Input: part model. Units: mm. Frame: model coordinates. Face numbers are marked on the shaded views. A direction names the side the tool comes from. Give positions to 0.01 mm unless a question says otherwise; leave off trailing zeros. Loops run counter-clockwise (first coordinate to the right, second up) from the corner with the lowest first, then second, coordinate; pieces in that order, holes last. Notation, with made-up numbers: M -19.5,-2 L 36.5,-2 A12 ccw 36.5,2 Z; hole C 26,-4.5 d9. An arc over 180 degrees is marked long. Answer as a JSON object with one key per item and string values. Group by question number.
1) Draft query along Z for the marked faces 1, 2, 3 and 4. Return one class per face: +Z half, -Z half, draft (parallel to the pull), parting line (faces both ways), or undercut.
2) Section query C-C on z = 1. Return loops of the section in (x, y), plus the area to 3 significant figures.
3) Section query D-D on y = 1.65. Return loops of the section in (x, z), plus the area to 3 significant figures.
4) Access query for the marked faces 5 and 6. Directions: +Z, -Z, +X, -X, +Y, -Y. A direction counts if a zero-diameter tool reaches every point of the face in a straight line with its end or side. Return the directions, or none.
5) First-contact query: P1, Ø1.5, axis at x = -3.5, y = 0.5, coming from the -Z side. Flat tip, straight axial feed; report the tip coordinate or a pass-through.
6) Section query A-A on x = 0. Return loops of the section in (y, z), plus the area to 3 significant figures.
7) Ray query, L1, parallel to Z at x = 0, y = 0.4; L2, parallel to Z at x = -5.5, y = 0; L3, parallel to X at y = 1.8, z = -32. Return the intervals inside material, ascending.
8) Section query B-B on x = 8.5. Return loops of the section in (y, z).
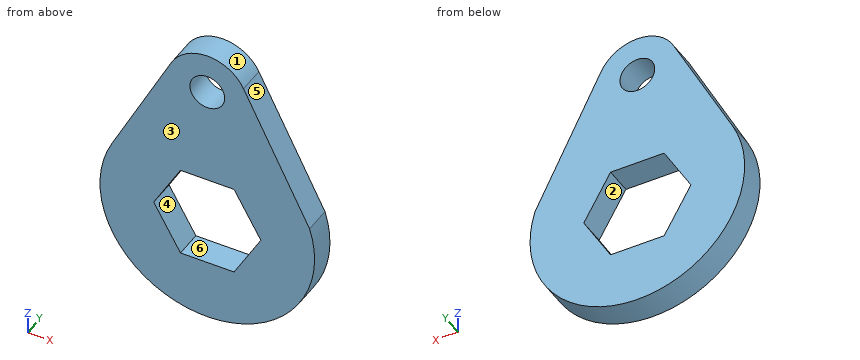
Autodesk Inventor part; units mm, degrees
ref_plane "YZ Plane" through (0, 0, 0) normal (1, 0, 0) x (0, 1, 0)
ref_plane "XZ Plane" through (0, 0, 0) normal (0, 1, 0) x (-1, 0, 0)
ref_plane "XY Plane" through (0, 0, 0) normal (0, 0, 1) x (1, 0, 0)
sketch "Sketch1" plane through (0, 0, 0) normal (0, 1, 0) x (-1, 0, 0)
  circle A0 centre (0, 0) radius 3
  circle A1 centre (0, 0) radius 7
  circle A2 centre (0, -25) radius 18.5
  line L0 (6.2154, 3.22) -> (16.4265, -16.49)
  line L1 (-17.6376, -19.4175) -> (-6.2496, 3.1532)
  line L2 (9.2376, -25) -> (4.6188, -33)
  line L3 (4.6188, -33) -> (-4.6188, -33)
  line L4 (-4.6188, -33) -> (-9.2376, -25)
  line L5 (-9.2376, -25) -> (-4.6188, -17)
  line L6 (-4.6188, -17) -> (4.6188, -17)
  line L7 (4.6188, -17) -> (9.2376, -25)
  point P0 (4.4139, 5.433)
  point P1 (-13.2255, -12.0641)
  dimension "d3" = 6
  dimension "d6" = 14
  dimension "d11" = 25
  dimension "d12" = 37
  dimension "d13" = 16
extrude "Plate1" add sketch "Sketch1" along normal mid plane 4.7 contours A1 A2 | A1 L0 A2 | A2 L1 A1 | A1 A2 | A1 A2 L1
equation "\"d9\" = Thickness"
equation "\"BendRadius\" = Thickness"
equation "\"BendReliefWidth\" = Thickness"
equation "\"BendReliefDepth\" = 0.5 * Thickness"
equation "\"CornerReliefSize\" = 4 * Thickness"
equation "\"MinimumRemnant\" = 2 * Thickness"
equation "\"TransitionRadius\" = BendRadius"
equation "\"JacobiRadiusSize\" = BendRadius"
equation "\"GapSize\" = Thickness"
properties part number "palanca2"
Output:
{
 "1": {"face 1": "+Z half", "face 2": "undercut", "face 3": "draft", "face 4": "undercut"},
 "2": {"outline": "M -7.37,-2.35 L -2.83,-2.35 L -2.83,2.35 L -7.37,2.35 Z; M 2.83,-2.35 L 7.34,-2.35 L 7.34,2.35 L 2.83,2.35 Z", "area": "42.5 mm^2"},
 "3": {"outline": "M -16.43,-16.49 A18.5 ccw long 17.64,-19.42 L 6.25,3.15 A7 ccw -6.22,3.22 Z; hole M -9.24,-25 L -4.62,-33 L 4.62,-33 L 9.24,-25 L 4.62,-17 L -4.62,-17 Z; hole C 0,0 d6", "area": "1,070 mm^2"},
 "4": {"face 5": "+Z, +X, +Y, -Y", "face 6": "+Y, -Y"},
 "5": {"P1": "stops at z = -43.29"},
 "6": {"outline": "M -2.35,-43.5 L 2.35,-43.5 L 2.35,-33 L -2.35,-33 Z; M -2.35,-17 L 2.35,-17 L 2.35,-3 L -2.35,-3 Z; M -2.35,3 L 2.35,3 L 2.35,7 L -2.35,7 Z", "area": "134 mm^2"},
 "7": {"L1": "z = -43.5 to -33, -17 to -3, 3 to 7", "L2": "z = -42.66 to -31.47, -18.53 to 4.33", "L3": "x = -17.12 to -5.2, 5.2 to 17.12"},
 "8": {"outline": "M -2.35,-41.43 L 2.35,-41.43 L 2.35,-26.28 L -2.35,-26.28 Z; M -2.35,-23.72 L 2.35,-23.72 L 2.35,-1.31 L -2.35,-1.31 Z"}
}
